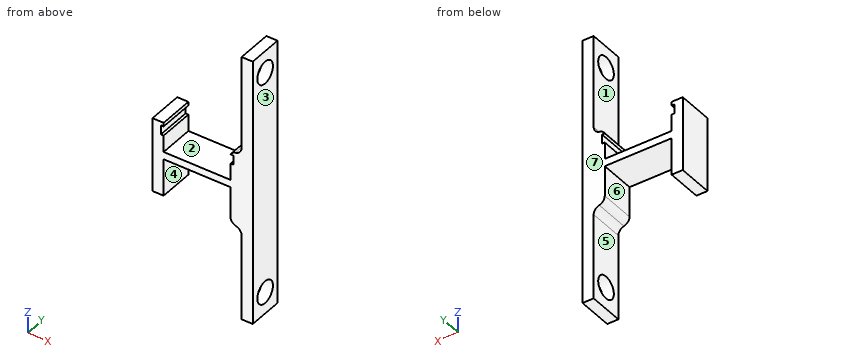
Autodesk Inventor part; units mm, degrees
ref_plane "YZ Plane" through (0, 0, 0) normal (1, 0, 0) x (0, 1, 0)
ref_plane "XZ Plane" through (0, 0, 0) normal (0, 1, 0) x (-1, 0, 0)
ref_plane "XY Plane" through (0, 0, 0) normal (0, 0, 1) x (1, 0, 0)
sketch "Sketch1" plane through (0, 0, 0) normal (0, 1, 0) x (-1, 0, 0)
  line L0 (-3.0388, 7.0833) -> (-6.0388, 7.0833)
  line L1 (-6.0388, 7.0833) -> (-6.0388, -12.9167)
  line L2 (-6.0388, -12.9167) -> (-3.0388, -12.9167)
  line L3 (-3.0388, -12.9167) -> (-3.0388, -2.9167)
  line L4 (-3.0388, -2.9167) -> (14.9612, -2.9167)
  line L5 (14.9612, -12.9167) -> (17.9612, -12.9167)
  line L6 (17.9612, -12.9167) -> (17.9612, 7.0833)
  line L7 (17.9612, 7.0833) -> (14.9612, 7.0833)
  line L8 (14.9612, 7.0833) -> (14.9612, 6.0833)
  line L9 (14.9612, 6.0833) -> (15.7112, 6.0833)
  line L10 (15.7112, 6.0833) -> (15.7112, 3.5833)
  line L11 (15.7112, 3.5833) -> (14.9612, 3.5833)
  line L12 (14.9612, 3.5833) -> (14.9612, -0.9167)
  line L13 (14.9612, -0.9167) -> (-3.0388, -0.9167)
  line L14 (-3.0388, -0.9167) -> (-3.0388, 3.5833)
  line L15 (-3.7888, 3.5833) -> (-3.7888, 6.0833)
  line L16 (-3.7888, 6.0833) -> (-3.0388, 6.0833)
  line L17 (-3.0388, 3.5833) -> (-3.7888, 3.5833)
  line L18 (-3.0388, 6.0833) -> (-3.0388, 7.0833)
  line L19 (14.9612, -12.9167) -> (14.9612, -2.9167)
  line L20 (-6.0388, 7.0833) -> (-6.0388, 34.0833)
  line L21 (-6.0388, 34.0833) -> (-9.0388, 34.0833)
  line L22 (-9.0388, 34.0833) -> (-9.0388, -37.9167)
  line L23 (-9.0388, -37.9167) -> (-6.0388, -37.9167)
  line L24 (-6.0388, -37.9167) -> (-6.0388, -12.9167)
  point P0 (0, 0)
  point P1 (14.9612, 1.3333)
  dimension "d0" = 2.5
  dimension "d1" = 3
  dimension "d2" = 3
  dimension "d3" = 10
  dimension "d4" = 10
  dimension "d5" = 2
  dimension "d6" = 3
  dimension "d8" = 1
  dimension "d9" = 8
  dimension "d11" = 0.75
  dimension "d12" = 0.75
  dimension "d13" = 3
  dimension "d16" = 18
  dimension "d17" = 3
  dimension "d18" = 72
  dimension "d19" = 35
extrude "Extrusion1" add sketch "Sketch1" along normal blind 9.5
fillet "Fillet1" radius 2 4 edges at (6.0388, 4.75, 7.0833) (6.0388, 4.75, -12.9167) (3.0388, 4.75, -12.9167) (3.0388, 4.75, 7.0833)
sketch "Sketch2" plane through (6.0388, 0, 34.0833) normal (-1, 0, 0) x (0, 0, 1)
  circle A0 centre (-5.875, 4.75) radius 3
  circle A1 centre (-66.125, 4.75) radius 3
  line L0 (-72, 0) -> (-49, 0)
  line L1 (-72, 9.5) -> (-49, 9.5)
  line L2 (-25, 9.5) -> (0, 9.5)
  line L3 (0, 0) -> (0, 9.5)
  line L4 (-72, 0) -> (-72, 9.5)
  point P0 (-34.0833, 0)
  dimension "d21" = 6
  dimension "d22" = 6
  dimension "d23" = 9.5
  dimension "d24" = 4.75
  dimension "d25" = 4.75
  dimension "d26" = 60.25
  dimension "d27" = 72
  dimension "d28" = 5.875
extrude "Extrusion2" cut sketch "Sketch2" against normal through all
equation "\"d2\" = d1"
equation "\"d4\" = d3"
equation "\"d6\" = d2"
equation "\"d12\" = d11"
equation "\"d13\" = d1"
equation "\"d19\" = -0.5 * d5 + 0.5 * d18"
equation "\"d24\" = 0.5 * d23"
equation "\"d25\" = 0.5 * d23"
equation "\"d28\" = -0.5 * d26 + 0.5 * d27"
properties part number "CO-1-02-stepperControllerMount"
Verification items for the finished model (mm, model axes). Face numbers are marked on the shaded views. A direction names the side the tool comes from. Coordinates: 2 decimals unless noted, no trailing zeros. Order: outer loops, then holes, each group sorted by start corner. A loop starts at its lowest first (then second) coordinate and runs counter-clockwise, first axis right, second up. Notation, with made-up numbers: (-25, 2.25) -> (8, 2.25) arc R12 cw to (8, 9.25) -> close; hole circle Ø4 at (83.5, 63). An arc over 180 degrees is marked (long way). Put each result on its own line as item: value. Start each with the question number.
1. Mould release check, pull along X, two halves, no side actions. Record for the marked faces 5, 6 and 7: released by +X, released by -X, zero draft, split by the parting line, or undercut.
2. Cross-section at C-C, the plane x = 1.5. Record the boundary of the cut face in (y, z), then the cut area to 3 significant figures.
3. Cross-section at B-B, the plane y = 8.5. Record the boundary of the cut face in (x, z), then the cut area to 3 significant figures.
4. Go/stop test with flat-tipped pins: pin 1 Ø1.5 at (x, y) = (-17, 6) entering from +Z; pin 2 Ø0.6 at (x, y) = (-15.5, 6) entering from -Z; pin 3 Ø1 at (x, y) = (-5.5, 4.5) entering from -Z. Record where each tip stops, or that it passes through.
5. Cross-section at A-A, the plane y = 4.75. Count the separate pieces of the cut face and the enclosed holes in it, then the cut area to 3 significant figures.
6. Cross-section at D-D, the plane z = -18. Record the boundary of the cut face in (x, y), then the cut area to 3 significant figures.
7. Access from +Z, -Z, +X, -X, +Y, -Y to the whole of each face (thin tool, end or side, straight path). Record for the marked faces 1, 2, 3 and 4.
8. Material ranges on L1, parallel to X at y = 2, z = 1; L2, parallel to X at y = 3.75, z = 6; L3, parallel to Z at x = -1, y = 8, recorded low to high. Write a range as [from, to].
Computed:
1. face 5: released by -X
1. face 6: undercut
1. face 7: zero draft
2. outline: (0, -2.92) -> (9.5, -2.92) -> (9.5, -0.92) -> (0, -0.92) -> close
2. area: 19.0 mm2
3. outline: (-17.96, -12.92) -> (-14.96, -12.92) -> (-14.96, -2.92) -> (3.04, -2.92) -> (3.04, -11.04) arc R2 ccw to (4.54, -12.98) arc R2 cw to (6.04, -14.92) -> (6.04, -37.92) -> (9.04, -37.92) -> (9.04, 34.08) -> (6.04, 34.08) -> (6.04, 9.08) arc R2 cw to (4.43, 7.12) arc R2 ccw to (3.04, 6.08) -> (3.79, 6.08) -> (3.79, 3.58) -> (3.04, 3.58) -> (3.04, -0.92) -> (-14.96, -0.92) -> (-14.96, 3.58) -> (-15.71, 3.58) -> (-15.71, 6.08) -> (-14.96, 6.08) -> (-14.96, 7.08) -> (-17.96, 7.08) -> close
3. area: 369 mm2
4. pin 1: z = 7.08
4. pin 2: z = -12.92
4. pin 3: z = -2.92
5. separate pieces: 3
5. enclosed holes: 0
5. area: 333 mm2
6. outline: (6.04, 0) -> (9.04, 0) -> (9.04, 9.5) -> (6.04, 9.5) -> close
6. area: 28.5 mm2
7. face 1: +Z, -X, +Y, -Y
7. face 2: +Z, +Y, -Y
7. face 3: +Z, -Z, +X, +Y, -Y
7. face 4: -Z, +Y, -Y
8. L1: [-17.96, -14.96], [3.04, 9.04]
8. L2: [-17.96, -15.71], [3.79, 9.04]
8. L3: [-2.92, -0.92]
